Verification items for the finished model (mm, model axes). A direction names the side the tool comes from. Round coordinates to 2 decimals unless told otherwise and drop trailing zeros. Write each loop counter-clockwise with the first axis right and the second up, starting at its lowest first coordinate (ties: lowest second). Pieces come first, ordered by that corner, then holes. Notation, with made-up numbers: (16, -21.5) - (35, -21.5) arc R30 ccw to (35, 15.5) - close; hole circle Ø1 at (60.5, 41.5). An arc over 180 degrees is marked (long way). Answer as a JSON object with one key per item and string values.
```python
from build123d import *

# Parameters (mm, degrees)
SKETCH1_W               = 101.6
SKETCH1_H               = 53.4162
BOSS_EXTRUDE1_DEPTH     = 1.651
CHAMFER3_SIZE           = 3.556
CUT_EXTRUDE4_REACH      = 3.651
CUT_EXTRUDE5_REACH      = 3.651
SKETCH22_R              = 1.5621
ESQUISSE1_W             = 1.651
ESQUISSE1_H             = 53.4162
ENL_V_MAT_EXTRU_1_DEPTH = 20.32


with BuildPart() as part:
    # Sketch1 → Boss-Extrude1 (new body)
    with BuildSketch(Plane.XY):
        Rectangle(SKETCH1_W, SKETCH1_H)
    extrude(amount=BOSS_EXTRUDE1_DEPTH)

    # Chamfer3
    chamfer3_edges = [part.edges().sort_by_distance(p)[0] for p in [
        (-50.8, -26.7081, 0.8255),
    ]]
    chamfer(chamfer3_edges, length=CHAMFER3_SIZE)

    # Sketch13 → Cut-Extrude4 (cut, up to next)
    with BuildSketch(Plane(origin=(0, 0, 0), x_dir=(-1, 0, 0), z_dir=(0, 0, -1)), mode=Mode.PRIVATE) as cut_extrude4_sk1:
        Polygon((48.26, 24.9446647), (48.26, 14.0081), (50.8, 11.4681), (50.8, 26.7081), (46.4965647, 26.7081), align=None)
    cut_extrude4_tool1 = extrude(cut_extrude4_sk1.sketch, amount=-CUT_EXTRUDE4_REACH, mode=Mode.PRIVATE) & part.part
    add(cut_extrude4_tool1.solids().sort_by_distance((-49.48888, 19.973214, 0))[0], mode=Mode.SUBTRACT)

    # Sketch22 → Cut-Extrude5 (cut, up to next)
    with BuildSketch(Plane(origin=(0, 0, 0), x_dir=(-1, 0, 0), z_dir=(0, 0, -1)), mode=Mode.PRIVATE) as cut_extrude5_sk1:
        with Locations((38.4556, 24.1681)):
            Circle(SKETCH22_R)
    cut_extrude5_tool1 = extrude(cut_extrude5_sk1.sketch, amount=-CUT_EXTRUDE5_REACH, mode=Mode.PRIVATE) & part.part
    add(cut_extrude5_tool1.solids().sort_by_distance((-38.4556, 24.1681, 0))[0], mode=Mode.SUBTRACT)
    # Sketch22 → Cut-Extrude5 (cut, up to next)
    with BuildSketch(Plane(origin=(0, 0, 0), x_dir=(-1, 0, 0), z_dir=(0, 0, -1)), mode=Mode.PRIVATE) as cut_extrude5_sk2:
        with Locations((45.9486, -24.1681)):
            Circle(SKETCH22_R)
    cut_extrude5_tool2 = extrude(cut_extrude5_sk2.sketch, amount=-CUT_EXTRUDE5_REACH, mode=Mode.PRIVATE) & part.part
    add(cut_extrude5_tool2.solids().sort_by_distance((-45.9486, -24.1681, 0))[0], mode=Mode.SUBTRACT)

    # Esquisse1 → Enlèv. mat.-Extru.1 (cut)
    with BuildSketch(Plane(origin=(50.8, 0, 0), x_dir=(0, 0, -1), z_dir=(1, 0, 0))):
        with Locations((-0.8255, 0)):
            Rectangle(ESQUISSE1_W, ESQUISSE1_H)
    extrude(amount=-ENL_V_MAT_EXTRU_1_DEPTH, mode=Mode.SUBTRACT)


solid = part.part
```
Q1. Gauge pin test, flat end, axial feed: P1, Ø0.8, axis at y = 19, z = 0.5, coming from the -X side. Record the tip position at first contact, or that the pin passes through.
Geometry check:
{"P1": "stops at x = -48.26"}
Q2. Section check A-A, the plane y = 21. Record the cut outline in (x, z).
Geometry check:
{"outline": "(-48.26, 0) - (30.48, 0) - (30.48, 1.65) - (-48.26, 1.65) - close"}
Q3. Material ranges on line 1 along X through (y, z) = (18, 0.15); line 2 along X through (y, z) = (13.5, 0.85), recorded low to high. Write a range as [from, to].
Geometry check:
{"line 1": "x = [-48.26, 30.48]", "line 2": "x = [-48.77, 30.48]"}
Q4. Set-up check for faces 5 (the flat face through (-49, -24.95, 0.81)), 6 (the flat face through (-48.26, 20, 1)): record each of +Z, -Z, +X, -X, +Y, -Y from which the full face is reachable in a straight line by a thin tool's end or side.
Geometry check:
{"face 5": "+Z, -Z, -X, -Y", "face 6": "+Z, -Z, -X, +Y"}
Q5. Release check for a two-part mould opening along Y. For faces 1 (the flat face through (30.48, 0, 1)), 2 (the flat face through (-47.366, 25.839, 0.814)), 3 (the cylindrical face through (-39.946, 24.637, 0.814)), 4 (the cylindrical face through (-47.44, -23.7, 0.81)) record: released by +Y, released by -Y, zero draft, split by the parting line, or undercut.
Geometry check:
{"face 1": "zero draft", "face 2": "released by +Y", "face 3": "undercut", "face 4": "undercut"}
